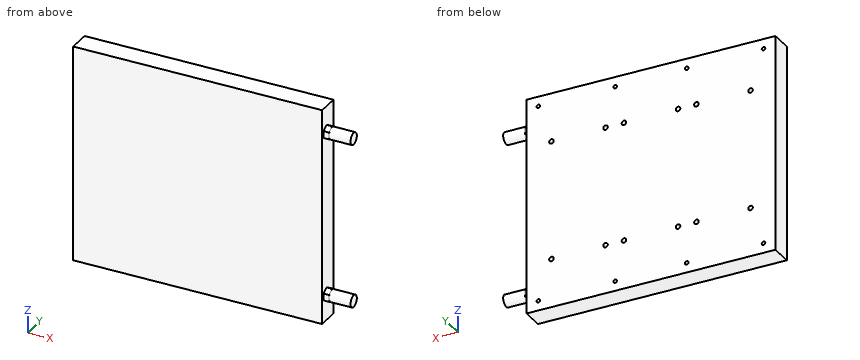
```python
from build123d import *

# Parameters (mm, degrees)
SZKIC1_W                    = 230
SZKIC1_H                    = 200
DODANIE_WYCI_GNI_CIE1_DEPTH = 20
OTW_R_GWINTOWANY_M52_D      = 4.2
OTW_R_GWINTOWANY_M52_DEPTH  = 14
OTW_R_GWINTOWANY_M52_TIP    = 1.2618073
OTW_R_GWINTOWANY_M41_D      = 3.3
OTW_R_GWINTOWANY_M41_DEPTH  = 11.5
OTW_R_GWINTOWANY_M41_TIP    = 0.991420021
DODANIE_WYCI_GNI_CIE2_DEPTH = 5
SZKIC10_R                   = 5.5
DODANIE_WYCI_GNI_CIE3_DEPTH = 20


with BuildPart() as part:
    # Szkic1 → Dodanie-wyciągnięcie1 (new body)
    with BuildSketch(Plane(origin=(0, 0, 0), x_dir=(1, 0, 0), z_dir=(0, 1, 0))):
        Rectangle(SZKIC1_W, SZKIC1_H)
    extrude(amount=DODANIE_WYCI_GNI_CIE1_DEPTH)

    # Otwór gwintowany M52
    with Locations(Plane(origin=(-92, 20, -55), x_dir=(0, 0, 1), z_dir=(0, 1, 0))):
        with Locations((0, 0), (0, 50), (0, 67), (0, 117), (110, 117), (110, 67), (110, 50), (110, 0), (110, 134), (0, 134), (0, 184), (110, 184)):
            Hole(OTW_R_GWINTOWANY_M52_D / 2, depth=OTW_R_GWINTOWANY_M52_DEPTH)
            with Locations((0, 0, -(OTW_R_GWINTOWANY_M52_DEPTH + OTW_R_GWINTOWANY_M52_TIP / 2))):  # 118° drill point
                Cone(0, OTW_R_GWINTOWANY_M52_D / 2, OTW_R_GWINTOWANY_M52_TIP, mode=Mode.SUBTRACT)

    # Otwór gwintowany M41
    with Locations(Plane(origin=(-104, 20, -91), x_dir=(0, 0, 1), z_dir=(0, 1, 0))):
        with Locations((0, 0), (0, 71), (0, 137), (0, 208), (182, 208), (182, 137), (182, 71), (182, 0)):
            Hole(OTW_R_GWINTOWANY_M41_D / 2, depth=OTW_R_GWINTOWANY_M41_DEPTH)
            with Locations((0, 0, -(OTW_R_GWINTOWANY_M41_DEPTH + OTW_R_GWINTOWANY_M41_TIP / 2))):  # 118° drill point
                Cone(0, OTW_R_GWINTOWANY_M41_D / 2, OTW_R_GWINTOWANY_M41_TIP, mode=Mode.SUBTRACT)

    # Szkic9 → Dodanie-wyciągnięcie2 (add)
    with BuildSketch(Plane(origin=(115, 0, 0), x_dir=(0, 0, -1), z_dir=(1, 0, 0))):
        Polygon((-69.649147039, 8), (-72.824573519, 13.5), (-79.175426481, 13.5), (-82.350852961, 8), (-79.175426481, 2.5), (-72.824573519, 2.5), align=None)
        Polygon((69.649147039, 8), (72.824573519, 2.5), (79.175426481, 2.5), (82.350852961, 8), (79.175426481, 13.5), (72.824573519, 13.5), align=None)
    extrude(amount=DODANIE_WYCI_GNI_CIE2_DEPTH)

    # Szkic10 → Dodanie-wyciągnięcie3 (add)
    with BuildSketch(Plane(origin=(120, 0, 0), x_dir=(0, 0, -1), z_dir=(1, 0, 0))):
        with Locations((76, 8)):
            Circle(SZKIC10_R)
        with Locations((-76, 8)):
            Circle(SZKIC10_R)
    extrude(amount=DODANIE_WYCI_GNI_CIE3_DEPTH)


solid = part.part
```
Read the model definition and answer for the solid it produces. Units are mm, in the model's axes. Round coordinates to 2 decimals unless told otherwise and drop trailing zeros. Write each loop counter-clockwise with the first axis right and the second up, starting at its lowest first coordinate (ties: lowest second). Pieces come first, ordered by that corner, then holes. Notation, with made-up numbers: (76.5, 42) - (128.5, 42) arc R13 cw to (128.5, 61) - close; hole circle Ø5 at (31, -16). An arc over 180 degrees is marked (long way). One line per item, written item: value.
Q1. Find section A-A (z = 9.5). Determine the outline of the cut face in (x, y).
The answers:
outline: (-115, 0) - (115, 0) - (115, 20) - (-115, 20) - close
Q2. Straight lines are drawn through the part: line 1 (Z direction, x = -42, y = 13); line 2 (Z direction, x = -33, y = 14); line 3 (X direction, y = 13.75, z = 91). For each, find the intervals that lie inside material, in ascending order. Write a range as from..to.
The answers:
line 1: z = -100..-57.1, -52.9..52.9, 57.1..100
line 2: z = -100..-92.65, -89.35..89.35, 92.65..100
line 3: x = -115..-105.65, -102.35..-34.65, -31.35..31.35, 34.65..102.35, 105.65..115
Q3. Each of these flat-tipped pins is pushed along its axis until it touches: P1, Ø1, axis at y = 9.5, z = -40, coming from the +X side; P2, Ø2.5, axis at x = 118, z = -76, coming from the +Y side; P3, Ø2.5, axis at x = 104, z = -91, coming from the +Y side. Where does it stop, or does it pass through?
The answers:
P1: stops at x = 115
P2: stops at y = 13.5
P3: stops at y = 8.26
